Can you work these out from the drawing? Everything is in mm from the part's minimum corner. Give positions to 0.01 mm unless a question says otherwise; leave off trailing zeros. Loops run counter-clockwise (first coordinate to the right, second up) from the corner with the lowest first, then second, coordinate; pieces in that order, holes last. Notation, with made-up numbers: (-6.5, 23) - (43.5, 23) arc R19 ccw to (43.5, 27) - close; hole circle Ø4 at (-13, 12.5). An arc over 180 degrees is marked (long way). Answer in a Markdown table with one row per item. Add a question column.
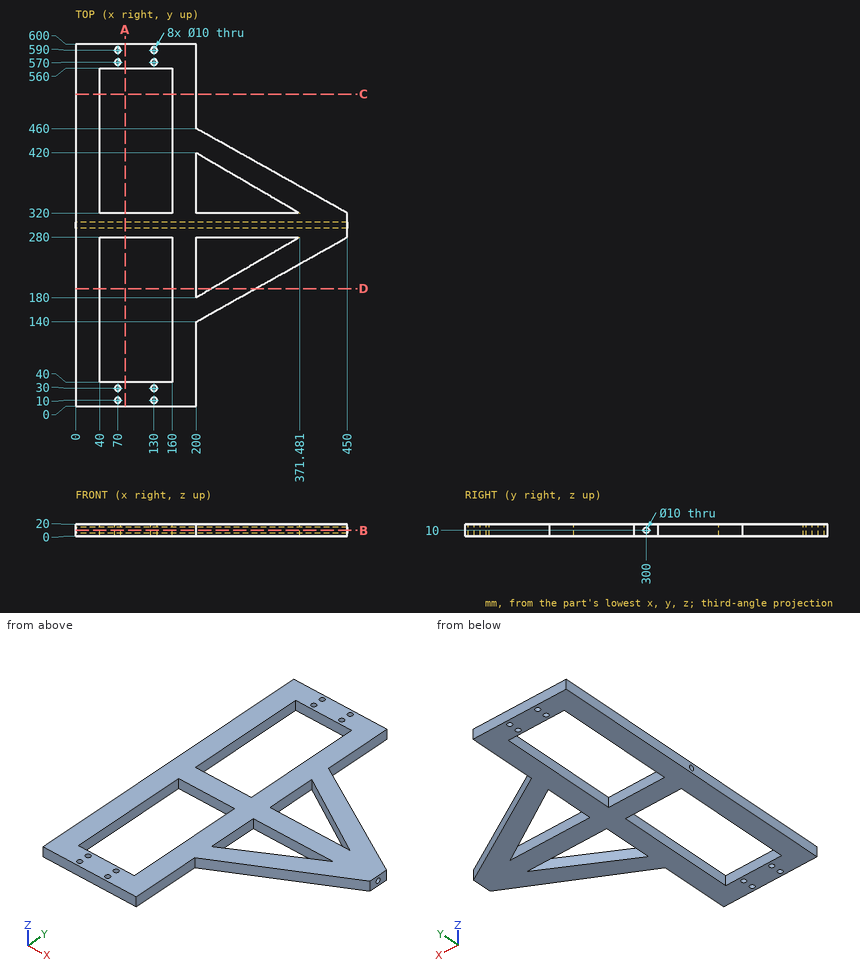
(1) I want a section at A-A on x = 82. Please give me the cut outline in (y, z), then the cut area to 3 significant figures.
(2) I want a section at B-B on z = 10. State how many separate pieces and enclosed holes the cut face has, then the cut area to 3 significant figures.
(3) For pin 1 Ø10 at (y, z) = (472.5, 7.5) entering from +X; pin 2 Ø10 at (x, z) = (246.5, 12) entering from +Y; pin 3 Ø1.5 at (x, z) = (239.5, 8.5) entering from -Y, each with a flat end and sliding along its axis, tell me the tip position at first contact or that it passes through.
(4) I want a section at C-C on y = 517. Please give me the cut outline in (x, z).
(5) Please list where these lines run through material, in increasing order: line 1 (X direction, y = 570, z = 9); line 2 (Y direction, x = 64, z = 18.5); line 3 (Z direction, x = 221, y = 300).
(6) I want a section at D-D on y = 195. Please give me the cut outline in (x, z).
Reported:
| question | item | result |
|---|---|---|
| 1 | outline | (0, 0) - (40, 0) - (40, 20) - (0, 20) - close; (280, 0) - (320, 0) - (320, 20) - (280, 20) - close; (560, 0) - (600, 0) - (600, 20) - (560, 20) - close; hole circle Ø10 at (300, 10) |
| 1 | area | 2,320 mm² |
| 2 | separate pieces | 2 |
| 2 | enclosed holes | 12 |
| 2 | area | 85,100 mm² |
| 3 | pin 1 | x = 200 |
| 3 | pin 2 | y = 436.76 |
| 3 | pin 3 | y = 161.7 |
| 4 | outline | (0, 0) - (40, 0) - (40, 20) - (0, 20) - close; (160, 0) - (200, 0) - (200, 20) - (160, 20) - close |
| 5 | line 1 | 0 to 65, 75 to 125, 135 to 200 |
| 5 | line 2 | 0 to 40, 280 to 320, 560 to 600 |
| 5 | line 3 | 0 to 5, 15 to 20 |
| 6 | outline | (0, 0) - (40, 0) - (40, 20) - (0, 20) - close; (160, 0) - (200, 0) - (200, 20) - (160, 20) - close; (225.72, 0) - (298.21, 0) - (298.21, 20) - (225.72, 20) - close |
